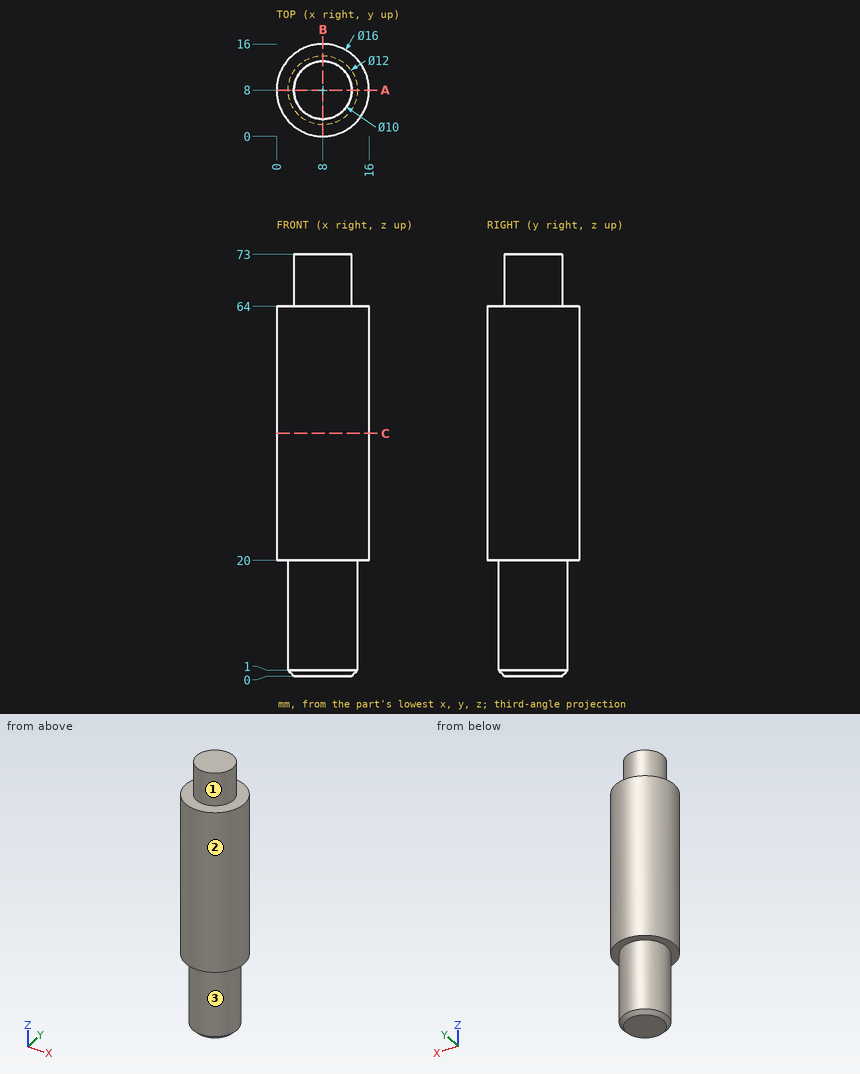
Check sheet for the drawn part. Datum: minimum x, y, z corner. Units: mm. A direction names the side the tool comes from. Round coordinates to 2 decimals unless told otherwise and drop trailing zeros. Order: outer loops, then holes, each group sorted by start corner. A loop starts at its lowest first (then second) coordinate and runs counter-clockwise, first axis right, second up.
1. Access from +Z, -Z, +X, -X, +Y, -Y to the whole of each face (thin tool, end or side, straight path). Record for the marked faces 1, 2 and 3.
Final values:
face 1: +Z
face 2: +Z, -Z
face 3: -Z
2. Thickness scan on L1, parallel to Z at x = 1.75, y = 11.25; L2, parallel to Y at x = 13, z = 34.5 (3 decimals); L3, parallel to Y at x = 5, z = 24. Record the ranges inside material, lowest first.
Final values:
L1: z = 20 to 64
L2: y = 1.755 to 14.245
L3: y = 0.58 to 15.42
3. Section check C-C on z = 42. Record the cut outline in (x, y).
Final values:
outline: circle Ø16 at (8, 8)
4. Section check A-A on y = 8. Record the cut outline in (x, z), then the cut area to 3 significant figures.
Final values:
outline: (0, 20) - (2, 20) - (2, 1) - (3, 0) - (13, 0) - (14, 1) - (14, 20) - (16, 20) - (16, 64) - (13, 64) - (13, 73) - (3, 73) - (3, 64) - (0, 64) - close
area: 1,030 mm2
5. Go/stop test with flat-tipped pins: P1, Ø1.5, axis at y = 11, z = 52, coming from the -X side; P2, Ø1.5, axis at x = 12, y = 2, coming from the -Z side; P3, Ø6, axis at y = 13, z = 65, coming from the +X side. Record where each tip stops, or that it passes through.
Final values:
P1: stops at x = 0.32
P2: stops at z = 20
P3: stops at x = 15.7
